The listing builds one solid part. Answer for the finished solid, in the listing's coordinates (mm). Give positions to 0.01 mm unless a question says otherwise; leave off trailing zeros. Loops run counter-clockwise (first coordinate to the right, second up) from the corner with the lowest first, then second, coordinate; pieces in that order, holes last. Notation, with made-up numbers: M 12,0.25 L 29,0.25 A18 ccw 29,16.25 Z; hole C 30,44.5 d11. An arc over 180 degrees is marked long. One line per item, written item: value. Start each with the question number.
Q1. A cutting plane is placed at C-C, the plane x = 21. Determine the outline of the cut face in (y, z).
Q2. Flat-ended cylindrical pins translate along their axes: pin 1 (1.5 mm diameter, centred on y = -36.5, z = 10, fed in from -X); pin 2 (6 mm diameter, centred on y = 54, z = 10.5, fed in from -X). Find the tip coordinate at first contact, or state that the pin passes through.
Q3. A cutting plane is placed at B-B, the plane y = 37. Determine the outline of the cut face in (x, z), and give its area (3 significant figures).
Q4. Consider L1, parallel to X at y = -61, z = 9.25; L2, parallel to X at y = -41.5, z = 11.5 (3 decimals); L3, parallel to Y at x = 21.5, z = 12. Determine where each line is inside the solid, lowest interval first.
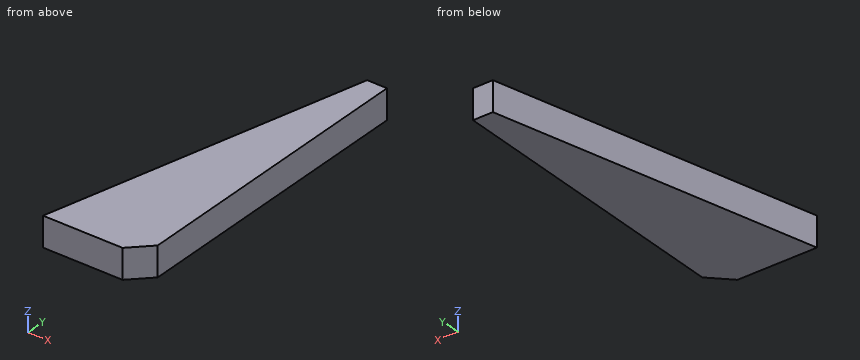
from build123d import *

# Parameters (mm, degrees)
F0_W     = 50
F0_H     = 160
F1_DEPTH = 15
F2_SIZE2 = 159.99999
F2_SIZE  = 39.99999
F3_SIZE2 = 10
F3_SIZE  = 10


# Not quite as in the source:
# - a fillet or chamfer is up to 0.001 mm smaller than in the source, because OpenCascade refuses the exact size


with BuildPart() as f1:
    # F0 (on Top) → F1 (new body)
    with BuildSketch(Plane.XY):
        Rectangle(F0_W, F0_H)
    extrude(amount=F1_DEPTH)

    # F2 (size 40 and 160 in the source; OpenCascade refuses exactly that, so slightly less here)
    f2_edges = [f1.edges().sort_by_distance(p)[0] for p in [
        (-25, 80, 7.5),
    ]]
    f2_side = f1.faces().sort_by_distance((0, 80, 7.5))[0]
    chamfer(f2_edges, length=F2_SIZE, length2=F2_SIZE2, reference=f2_side)

    # F3
    f3_edges = [f1.edges().sort_by_distance(p)[0] for p in [
        (25, -80, 7.5),
    ]]
    chamfer(f3_edges, length=F3_SIZE, length2=F3_SIZE2)


solid = f1.part
Answer block:
1. outline: M -74,0 L 80,0 L 80,15 L -74,15 Z
2. pin 1: x = -14.31
2. pin 2: x = 7.75
3. outline: M 4.25,0 L 25,0 L 25,15 L 4.25,15 Z
3. area: 311 mm^2
4. L1: -20.25 to 25
4. L2: -15.375 to 25
4. L3: -73.5 to 80
